Geometry: final body of the model. Coordinates: model frame, mm. A direction names the side the tool comes from. Give positions to 0.01 mm unless a question says otherwise; leave off trailing zeros. Write each loop counter-clockwise with the first axis right and the second up, starting at its lowest first coordinate (ties: lowest second). Pieces come first, ordered by that corner, then holes.
Q1. Cut plane D-D on y = -4.75. Return the cut outline in (x, z), plus the area to 3 significant figures.
Q2. Pin query (flat end, axial travel): pin 1 (2.5 mm diameter, centred on x = 10.34, z = 5.97, fed in from -Y); pin 2 (1.5 mm diameter, centred on y = 1, z = -4.5, fed in from +X); pin 3 (5 mm diameter, centred on y = -6, z = -8, fed in from -X); pin 4 (3 mm diameter, centred on y = 3, z = -4.5, fed in from +X). Return the tip coordinate at first contact, or that it passes through.
Q3. Cut plane A-A on z = 0. Return the cut outline in (x, y) (3 decimals), plus the area to 3 significant figures.
Q4. Cut plane C-C on y = 4.25. Count the separate pieces of the cut face and the enclosed holes in it, plus the area to 3 significant figures.
Q5. Draft query along X for faces 1 (the face through (-3.86, 4.78, -5.04)), 2 (the face through (11.913, 5.098, 5.762)), 3 (the face through (3.047, -5.653, 0.4)), 4 (the face through (3.3, 0, -3.3)). Return one class per face: pulls with the +X half, pulls with the -X half, needs draft (parallel to the pull), parting line crosses it, or undercut.
Q6. Reachability of faces 5 (the face through (15.11, 3.15, -1.98)), 6 (the face through (-0.966, 5.098, -13.198)) from +Z, -Z, +X, -X, +Y, -Y: full face, straight path, thin tool, end or side. Return the list, or none.
Q7. Line query: L1, parallel to Y at x = 8, z = -11; L2, parallel to Z at x = 3.5, y = 5.5; L3, parallel to X at y = 3.5, z = 2. Output: solid intervals per line, ascending.
```python
from build123d import *

# Parameters (mm, degrees)
SKETCH1_R           = 15.24
BOSS_EXTRUDE1_DEPTH = 6.35
SKETCH2_R           = 6.35
CUT_EXTRUDE1_DEPTH  = 3.175
FILLET4_R           = 1.27
SKETCH3_R           = 3.0734
BOSS_EXTRUDE3_DEPTH = 11.43
FILLET5_R           = 1.27
SKETCH4_R           = 1.5875
CUT_EXTRUDE2_DEPTH  = 2.54
CIRPATTERN1_COUNT   = 3


with BuildPart() as part:
    # Sketch1 → Boss-Extrude1 (new body)
    with BuildSketch(Plane(origin=(0, 0, 0), x_dir=(1, 0, 0), z_dir=(0, 1, 0))):
        with Locations(Location((0, 0, 0), (0, 0, 270))):
            Circle(SKETCH1_R)
    extrude(amount=BOSS_EXTRUDE1_DEPTH)

    # Sketch2 → Cut-Extrude1 (cut)
    with BuildSketch(Plane(origin=(0, 6.35, 0), x_dir=(1, 0, 0), z_dir=(0, 1, 0))):
        with Locations(Location((0, 0, 0), (0, 0, 270))):
            Circle(SKETCH2_R)
    extrude(amount=-CUT_EXTRUDE1_DEPTH, mode=Mode.SUBTRACT)

    # Fillet4
    fillet4_edges = [part.edges().sort_by_distance(p)[0] for p in [
        (0, 6.35, -15.24),
    ]]
    fillet(fillet4_edges, radius=FILLET4_R)

    # Sketch3 → Boss-Extrude3 (add)
    with BuildSketch(Plane.XZ):
        with Locations(Location((0, 0, 0), (0, 0, 270))):
            Circle(SKETCH3_R)
    extrude(amount=BOSS_EXTRUDE3_DEPTH)

    # Fillet5
    fillet5_edges = [part.edges().sort_by_distance(p)[0] for p in [
        (0, 0, 3.0734),
        (0, -11.43, 3.0734),
        (0, 0, -15.24),
    ]]
    fillet(fillet5_edges, radius=FILLET5_R)

    # Sketch4 → Cut-Extrude2 (cut)
    with BuildSketch(Plane(origin=(0, 6.35, 0), x_dir=(1, 0, 0), z_dir=(0, 1, 0))):
        with Locations(Location((0, 11.938, 0), (0, 0, 270))):
            Circle(SKETCH4_R)
    cut_extrude2 = extrude(amount=-CUT_EXTRUDE2_DEPTH, mode=Mode.SUBTRACT)

    # CirPattern1: Cut-Extrude2 ×3 about axis
    cirpattern1_axis = Axis((0, 0, 0), (0, 1, 0))
    for i in range(1, CIRPATTERN1_COUNT):
        add(cut_extrude2.rotate(cirpattern1_axis, i * 360 / CIRPATTERN1_COUNT), mode=Mode.SUBTRACT)


solid = part.part
```
Data:
1. outline: circle Ø6.15 at (0, 0)
1. area: 29.7 mm2
2. pin 1: stops at y = 0
2. pin 2: stops at x = 14.76
2. pin 3: passes through
2. pin 4: stops at x = 14.94
3. outline: (-15.24, 1.27) arc R1.27 ccw to (-13.97, 0) - (-4.343, 0) arc R1.27 cw to (-3.073, -1.27) - (-3.073, -10.16) arc R1.27 ccw to (-1.803, -11.43) - (1.803, -11.43) arc R1.27 ccw to (3.073, -10.16) - (3.073, -1.27) arc R1.27 cw to (4.343, 0) - (13.97, 0) arc R1.27 ccw to (15.24, 1.27) - (15.24, 5.08) arc R1.27 ccw to (13.97, 6.35) - (6.35, 6.35) - (6.35, 3.175) - (-6.35, 3.175) - (-6.35, 6.35) - (-13.97, 6.35) arc R1.27 ccw to (-15.24, 5.08) - close
3. area: 222 mm2
4. separate pieces: 1
4. enclosed holes: 4
4. area: 579 mm2
5. face 1: undercut
5. face 2: undercut
5. face 3: parting line crosses it
5. face 4: needs draft
6. face 5: +Y, -Y
6. face 6: +Y
7. L1: y = 0 to 6.35
7. L2: z = -14.76 to -5.3, 5.3 to 14.76
7. L3: x = -15.11 to -6.03, 6.03 to 15.11
